from build123d import *

# Parameters (mm, degrees)
SKICA1_R                = 7.5
SKICA1_R_2              = 5.25
P_IDAT_VYSUNUT_M1_DEPTH = 10
P_IDAT_START            = -2
SKICA1_3_R              = 10
SKICA1_3_R_2            = 7.5
SKICA1_3_R_3            = 5.25
P_IDAT_VYSUNUT_M2_DEPTH = 2
ZAOBLIT1_R              = 0.5


with BuildPart() as part:
    # Skica1 → P_idat vysunut_m1 (new body)
    with BuildSketch(Plane.XY):
        Circle(SKICA1_R)
        Circle(SKICA1_R_2, mode=Mode.SUBTRACT)
    extrude(amount=P_IDAT_VYSUNUT_M1_DEPTH)

    # Skica1_3 → P_idat vysunut_m2 (add)
    # profile 1 of 2: a face of its own
    with BuildSketch(Plane.XY.offset(P_IDAT_START)):
        Circle(SKICA1_3_R)
        Circle(SKICA1_3_R_2, mode=Mode.SUBTRACT)
    # profile 2 of 2: a face of its own
    with BuildSketch(Plane.XY.offset(P_IDAT_START)):
        Circle(SKICA1_3_R_2)
        Circle(SKICA1_3_R_3, mode=Mode.SUBTRACT)
    extrude(amount=P_IDAT_VYSUNUT_M2_DEPTH)

    # Zaoblit1
    zaoblit1_edges = [part.edges().sort_by_distance(p)[0] for p in [
        (-7.5, 0, 10),
        (-5.25, 0, 10),
        (-10, 0, -2),
        (-5.25, 0, -2),
    ]]
    fillet(zaoblit1_edges, radius=ZAOBLIT1_R)


solid = part.part
Input: part model. Units: mm. Frame: model coordinates. A direction names the side the tool comes from. Coordinates: 2 decimals unless noted, no trailing zeros. Order: outer loops, then holes, each group sorted by start corner. A loop starts at its lowest first (then second) coordinate and runs counter-clockwise, first axis right, second up.
1. Draft query along X for faces 1 (the cylindrical face through (-2.17, -9.76, -0.76)), 2 (the flat face through (-1, 6, 10)), 3 (the cylindrical face through (5, 1.6, 3.9)). Return one class per face: +X half, -X half, draft (parallel to the pull), parting line (faces both ways), or undercut.
Checked values:
face 1: parting line
face 2: draft
face 3: undercut
2. Access query for faces 4 (the cylindrical face through (-7.493, 0.33, 4.684)), 5 (the flat face through (0, -6, -2)). Directions: +Z, -Z, +X, -X, +Y, -Y. A direction counts if a zero-diameter tool reaches every point of the face in a straight line with its end or side. Return the directions, or none.
Checked values:
face 4: +Z
face 5: -Z, +X, -X, +Y, -Y
3. Cut plane C-C, the plane z = 2.25. Return loops of the section in (x, y).
Checked values:
outline: circle Ø15 at (0, 0); hole circle Ø10.5 at (0, 0)
4. Cut plane A-A, the plane x = 0. Return loops of the section in (y, z).
Checked values:
outline: (-10, -1.5) arc R0.5 ccw to (-9.5, -2) - (-5.75, -2) arc R0.5 ccw to (-5.25, -1.5) - (-5.25, 9.5) arc R0.5 ccw to (-5.75, 10) - (-7, 10) arc R0.5 ccw to (-7.5, 9.5) - (-7.5, 0) - (-10, 0) - close; (5.25, -1.5) arc R0.5 ccw to (5.75, -2) - (9.5, -2) arc R0.5 ccw to (10, -1.5) - (10, 0) - (7.5, 0) - (7.5, 9.5) arc R0.5 ccw to (7, 10) - (5.75, 10) arc R0.5 ccw to (5.25, 9.5) - close
5. Ray query, line 1 along Y through (x, z) = (0, 2.25); line 2 along Z through (x, y) = (-3.75, 8.5); line 3 along Z through (x, y) = (6.5, -2.75). Return the intervals inside material, ascending.
Checked values:
line 1: y = -7.5 to -5.25, 5.25 to 7.5
line 2: z = -2 to 0
line 3: z = -2 to 10
6. Contact query for flat-ended pins moving along their axis: P1, Ø5, axis at x = 2.5, z = 8, coming from the -Y side; P2, Ø1.5, axis at y = 2, z = 5.5, coming from the +X side; P3, Ø2, axis at y = -4, z = 8, coming from the +X side; P4, Ø8.5, axis at x = 0, y = 0, coming from the +Z side. Output: stop coordinate, or through.
Checked values:
P1: stops at y = -7.5
P2: stops at x = 7.4
P3: stops at x = 6.87
P4: passes through
